Build history of the part. All positions in model axes, mm. A direction names the side the tool comes from. Coordinates: 2 decimals unless noted, no trailing zeros. Order: outer loops, then holes, each group sorted by start corner. A loop starts at its lowest first (then second) coordinate and runs counter-clockwise, first axis right, second up. Notation, with made-up numbers: (62.25, 21.25) -> (90.25, 21.25) arc R29 cw to (90.25, 44.25) -> close; hole circle Ø11 at (63, 61). An arc over 180 degrees is marked (long way). Write each question's results on one line, items separated by ' | '.
from build123d import *

# Parameters (mm, degrees)
F1_DEPTH  = 426
F3_DEPTH  = 4
F4_R      = 2
F7_DEPTH  = 4
F10_DEPTH = 4


# Not quite as in the source:
# - a feature names something its author has since deleted; it is built from what else it names


with BuildPart() as f1:
    # F0 (on Top) → F1 (new body)
    with BuildSketch(Plane.XY):
        Polygon((-200, -343), (0, -343), (0, 0), (-495, 0), (-495, -1261), (-491, -1261), (-491, -4), (-4, -4), (-4, -339), (-204, -339), (-204, -1261), (-200, -1261), align=None)
    extrude(amount=F1_DEPTH)

    # F2 (on Top) → F3 (join)
    with BuildSketch(Plane.XY):
        Polygon((0, 0), (-495, 0), (-495, -1261), (-200, -1261), (-200, -343), (0, -343), align=None)
    extrude(amount=-F3_DEPTH)

    # F4
    f4_edges = [f1.edges().sort_by_distance(p)[0] for p in [
        (-200, -802, -4),
        (-495, -630.5, -4),
        (-247.5, 0, -4),
        (0, -343, 211),
        (0, 0, 211),
    ]]
    fillet(f4_edges, radius=F4_R)

    # F6 (on offset) → F7 (join)
    with BuildSketch(Plane.XZ.offset(961)):
        Polygon((-491, 355), (-491, 0), (-269, 0), align=None)
    extrude(amount=F7_DEPTH)

    # F9 (on offset) → F10 (join)
    with BuildSketch(Plane.XZ.offset(361)):
        Polygon((-426, 0), (-204, 0), (-204, 355), align=None)
    extrude(amount=F10_DEPTH)


solid = f1.part
Item 1: Drill centre lines: line 1 (Y direction, x = -378, z = 69); line 2 (Y direction, x = -434, z = 191); line 3 (Y direction, x = -224, z = 175). Where is each one in solid material? Low to high. Write a range as from..to.
Answer:
line 1: y = -965..-961, -365..-361, -4..0 | line 2: y = -965..-961, -4..0 | line 3: y = -365..-361, -4..0
Item 2: Slice it at A-A, the plane y = -112.5. List the corners of the cut face in (x, z).
Answer:
outline: (-495, -2) arc R2 ccw to (-493, -4) -> (0, -4) -> (0, 426) -> (-4, 426) -> (-4, 0) -> (-491, 0) -> (-491, 426) -> (-495, 426) -> close
Item 3: Slice it at C-C, the plane x = -336. List the corners of the cut face in (y, z), and give its area (3 significant figures).
Answer:
outline: (-1261, -4) -> (-2, -4) arc R2 ccw to (0, -2) -> (0, 426) -> (-4, 426) -> (-4, 0) -> (-361, 0) -> (-361, 143.92) -> (-365, 143.92) -> (-365, 0) -> (-961, 0) -> (-961, 107.14) -> (-965, 107.14) -> (-965, 0) -> (-1261, 0) -> close | area: 7,750 mm^2
Item 4: Slice it at D-D, the plane y = -1124. List the corners of the cut face in (x, z).
Answer:
outline: (-495, -2) arc R2 ccw to (-493, -4) -> (-202, -4) arc R2 ccw to (-200, -2) -> (-200, 426) -> (-204, 426) -> (-204, 0) -> (-491, 0) -> (-491, 426) -> (-495, 426) -> close
Item 5: Slice it at B-B, the plane z = 367.5. List the corners of the cut face in (x, y), and give its area (3 significant figures).
Answer:
outline: (-495, -1261) -> (-491, -1261) -> (-491, -4) -> (-4, -4) -> (-4, -339) -> (-204, -339) -> (-204, -1261) -> (-200, -1261) -> (-200, -343) -> (-2, -343) arc R2 ccw to (0, -341) -> (0, -2) arc R2 ccw to (-2, 0) -> (-495, 0) -> close | area: 12,800 mm^2
Item 6: Pin check, flat tips, straight feed: pin 1 (4 mm diameter, centred on x = -279, z = 320.5, fed in from -Y); pin 2 (1 mm diameter, centred on y = -787.5, z = 39, fed in from +X); pin 3 (1 mm diameter, centred on x = -325.5, y = -781.5, fed in from +Z). Stop position of each tip, or through.
Answer:
pin 1: stops at y = -4 | pin 2: stops at x = -200 | pin 3: stops at z = 0
Item 7: Tool access for faces 1 (the flat face through (0, -174, 214)), 2 (the flat face through (-251, -4, 210)), 3 (the flat face through (-103, -343, 214)): list every direction of +Z, -Z, +X, -X, +Y, -Y with a clear straight run to the whole face (end or side of a thin tool).
Answer:
face 1: +Z, -Z, +X, +Y, -Y | face 2: +Z | face 3: +Z, -Z, +X, -Y
Item 8: Pull direction Y, two halves, no side cores. Call faces 4 (the flat face through (-200, -808, 215)), 5 (the flat face through (-103, -339, 210)), 6 (the flat face through (-431, -965, 101)): released by +Y, released by -Y, zero draft, split by the parting line, or undercut.
Answer:
face 4: zero draft | face 5: undercut | face 6: released by -Y
